Design review of the part built by this model. Coordinates are the model's own, in mm. A direction names the side the tool comes from. Give positions to 0.01 mm unless a question says otherwise; leave off trailing zeros. Write each loop counter-clockwise with the first axis right and the second up, starting at its lowest first coordinate (ties: lowest second). Pieces come first, ordered by that corner, then holes. Notation, with made-up numbers: (14.25, 53) -> (37.25, 53) arc R23 cw to (37.25, 64) -> close; hole circle Ø7 at (-26.5, 23). An arc over 180 degrees is marked (long way). Answer as a JSON object with one key per item and string values.
```python
from build123d import *

# Parameters (mm, degrees)
F0_R     = 19.05
F1_DEPTH = 80
F4_R     = 19.05
F4_R_2   = 18.55
F5_DEPTH = 20
F3_W     = 27
F3_H     = 3
F6_DEPTH = 70
F8_W     = 34
F8_H     = 5
F9_DEPTH = 62


with BuildPart() as f1:
    # F0 (on Front) → F1 (new body)
    with BuildSketch(Plane.XZ):
        Circle(F0_R)
    extrude(amount=-F1_DEPTH)

    # F4 (on face) → F5 (join)
    with BuildSketch(Plane(origin=(0, 80, 0), x_dir=(-1, 0, 0), z_dir=(0, 1, 0))):
        Circle(F4_R)
        Circle(F4_R_2, mode=Mode.SUBTRACT)
    extrude(amount=F5_DEPTH)

    # F3 (on Front) → F6 (cut)
    with BuildSketch(Plane.XZ):
        with Locations((0, 9)):
            Rectangle(F3_W, F3_H)
        with Locations((0, -9)):
            Rectangle(F3_W, F3_H)
    extrude(amount=-F6_DEPTH, mode=Mode.SUBTRACT)

    # F8 (on Front) → F9 (cut)
    with BuildSketch(Plane.XZ):
        Rectangle(F8_W, F8_H)
    extrude(amount=-F9_DEPTH, mode=Mode.SUBTRACT)


solid = f1.part
```
(1) For line 1 along Z through (x, y) = (0, 86.5); line 2 along Z through (x, y) = (5.5, 42); line 3 along Z through (x, y) = (5, 15), list the stretches that pass through material, from the lowest coordinate up.
Here are the results:
{"line 1": "z = -19.05 to -18.55, 18.55 to 19.05", "line 2": "z = -18.24 to -10.5, -7.5 to -2.5, 2.5 to 7.5, 10.5 to 18.24", "line 3": "z = -18.38 to -10.5, -7.5 to -2.5, 2.5 to 7.5, 10.5 to 18.38"}
(2) We need section B-B, the plane z = 0. State the section outline as (x, y) points.
Here are the results:
{"outline": "(-19.05, 0) -> (-17, 0) -> (-17, 62) -> (17, 62) -> (17, 0) -> (19.05, 0) -> (19.05, 100) -> (18.55, 100) -> (18.55, 80) -> (-18.55, 80) -> (-18.55, 100) -> (-19.05, 100) -> close"}
(3) For faces 3 (the cylindrical face through (2.415, 89.86, 18.392)), 4 (the flat face through (13.5, 35, 9)), 5 (the flat face through (-4.1, 100, -18.3)), list the 3-axis set-ups (+Z, -Z, +X, -X, +Y, -Y) from which the entire face can be reached by the end or side of a thin tool; tool diameter is ignored.
Here are the results:
{"face 3": "+Y", "face 4": "-Y", "face 5": "+Z, -Z, +X, -X, +Y"}
(4) We need section A-A, the plane y = 29. State the section outline as (x, z) points.
Here are the results:
{"outline": "circle Ø38.1 at (0, 0); hole (-17, -2.5) -> (17, -2.5) -> (17, 2.5) -> (-17, 2.5) -> close; hole (-13.5, -10.5) -> (13.5, -10.5) -> (13.5, -7.5) -> (-13.5, -7.5) -> close; hole (-13.5, 7.5) -> (13.5, 7.5) -> (13.5, 10.5) -> (-13.5, 10.5) -> close"}
(5) We need section D-D, the plane y = 90. State the section outline as (x, z) points.
Here are the results:
{"outline": "circle Ø38.1 at (0, 0); hole circle Ø37.1 at (0, 0)"}
(6) Clearance check with flat-ended pins moving along their axes: pin 1 (3 mm diameter, centred on x = 11.5, z = -8, fed in from -Y); pin 2 (11 mm diameter, centred on x = 6.5, z = 7.5, fed in from +Y); pin 3 (21.5 mm diameter, centred on x = -3, y = 24.5, fed in from -Z); pin 4 (1.5 mm diameter, centred on y = 34, z = 9, fed in from +X). State where each tip first meets the part, or that it passes through.
Here are the results:
{"pin 1": "stops at y = 0", "pin 2": "stops at y = 80", "pin 3": "stops at z = -19.05", "pin 4": "stops at x = 17.17"}
(7) The part is to be moulded in two halves that separate along Z. For faces 1 (the flat face through (0, 0, -4)), 2 (the flat face through (0, 31, -2.5)), say which applies: +Z half, -Z half, draft (parallel to the pull), parting line (faces both ways), or undercut.
Here are the results:
{"face 1": "draft", "face 2": "undercut"}
(8) We need section C-C, the plane x = 0. State the section outline as (y, z) points, then the cut area to 3 significant figures.
Here are the results:
{"outline": "(0, -19.05) -> (100, -19.05) -> (100, -18.55) -> (80, -18.55) -> (80, 18.55) -> (100, 18.55) -> (100, 19.05) -> (0, 19.05) -> (0, 10.5) -> (70, 10.5) -> (70, 7.5) -> (0, 7.5) -> (0, 2.5) -> (62, 2.5) -> (62, -2.5) -> (0, -2.5) -> (0, -7.5) -> (70, -7.5) -> (70, -10.5) -> (0, -10.5) -> close", "area": "2,340 mm²"}
